Geometry check sheet. Reference: the model listing, model coordinates, mm. Face numbers are marked on the shaded views. A direction names the side the tool comes from. Give positions to 0.01 mm unless a question says otherwise; leave off trailing zeros. Write each loop counter-clockwise with the first axis right and the second up, starting at its lowest first coordinate (ties: lowest second). Pieces come first, ordered by that corner, then holes. Notation, with made-up numbers: (14.5, -34.75) -> (19.5, -34.75) arc R7 cw to (19.5, -22.75) -> close; hole circle Ø3 at (-30.75, 54.5). An arc over 180 degrees is marked (long way). Write item = value, one per line. Start each with the question number.
1. Depth check by flat-ended pin: P1, Ø6.5, axis at x = 325, z = -258.5, coming from the -Y side; P2, Ø11, axis at x = 292.5, z = 7.5, coming from the -Y side; P3, Ø8, axis at x = 92.5, z = 7.5, coming from the +Y side; P4, Ø1, axis at y = 1, z = 300.5, coming from the +X side. Enter the tip coordinate at first touch or a pass-through.
2. Thickness scan on line 1 along X through (y, z) = (1.4, -162.5); line 2 along Z through (x, y) = (-325, 1.55); line 3 along X through (y, z) = (-3.75, 85). Record the ranges inside material, lowest first.
3. Cross-section at B-B, the plane z = -92. Record the cut outline in (x, y).
4. Set-up check for the marked faces 1 and 2: record each of +Z, -Z, +X, -X, +Y, -Y from which the full face is reachable in a straight line by a thin tool's end or side.
5. Cross-section at A-A, the plane y = -6.25. Record the cut outline in (x, z).
6. Cross-section at C-C, the plane x = -145.5. Record the cut outline in (y, z), plus the area to 3 significant figures.
```python
from build123d import *

# Parameters (mm, degrees)
SM_BASE_FLANGE_1_DEPTH = 308.5
SKETCH_6_W             = 10
SKETCH_6_H             = 10
CUT_EXTRUDE_1_DEPTH    = 474.827500257
OTHER_1_DEPTH          = 2
SKETCH_7_R             = 5.5
CUT_EXTRUDE_2_DEPTH    = 10
SKETCH_8_R             = 3.5
CUT_EXTRUDE_3_DEPTH    = 10


# Read off the part's stored shape, not the designer's step: Затупленный угол1
# Sheet-metal steps are written as plain solids
with BuildPart() as part:
    # Sketch 1 → Базовая кромка1 (new, symmetric)
    with BuildSketch(Plane.XY):
        with BuildLine():
            Line((-357.5, -8), (-357.5, -2))
            ThreePointArc((-357.5, -2), (-356.914213562, -0.585786438), (-355.5, 0))
            Line((-355.5, 0), (355.5, 0))
            ThreePointArc((355.5, 0), (356.914213562, -0.585786438), (357.5, -2))
            Line((357.5, -2), (357.5, -8))
            Line((357.5, -8), (359.5, -8))
            Line((359.5, -8), (359.5, -2))
            ThreePointArc((359.5, -2), (358.328427125, 0.828427125), (355.5, 2))
            Line((355.5, 2), (-355.5, 2))
            ThreePointArc((-355.5, 2), (-358.328427125, 0.828427125), (-359.5, -2))
            Line((-359.5, -2), (-359.5, -8))
            Line((-359.5, -8), (-357.5, -8))
        make_face()
    extrude(amount=SM_BASE_FLANGE_1_DEPTH, both=True)

    # Эскиз6 → Вырез-Вытянуть1 (cut, through all)
    with BuildSketch(Plane(origin=(0, 2, 0), x_dir=(1, 0, 0), z_dir=(0, 1, 0))):
        with Locations((-354.5, -303.5)):
            Rectangle(SKETCH_6_W, SKETCH_6_H)
        with Locations((354.5, -303.5)):
            Rectangle(SKETCH_6_W, SKETCH_6_H)
    extrude(amount=-CUT_EXTRUDE_1_DEPTH, mode=Mode.SUBTRACT)

    # Other 1 outline → Other 1 (cut)
    with BuildSketch(Plane(origin=(0, 0, 0), x_dir=(1, 0, 0), z_dir=(0, 1, 0))):
        Polygon((-349.5, -308.5), (-344.5, -308.5), (-349.5, -303.5), align=None)
        Polygon((349.5, -303.5), (344.5, -308.5), (349.5, -308.5), align=None)
    extrude(amount=OTHER_1_DEPTH, mode=Mode.SUBTRACT)

    # Эскиз7 → Вырез-Вытянуть2 (cut)
    with BuildSketch(Plane(origin=(0, 2, 0), x_dir=(1, 0, 0), z_dir=(0, 1, 0))):
        with Locations(Location((325, -293.5, 0), (0, 0, 270))):
            Circle(SKETCH_7_R)
        with Locations(Location((-325, -293.5, 0), (0, 0, 270))):
            Circle(SKETCH_7_R)
        with Locations(Location((-325, 258.5, 0), (0, 0, 270))):
            Circle(SKETCH_7_R)
        with Locations(Location((325, 258.5, 0), (0, 0, 270))):
            Circle(SKETCH_7_R)
    extrude(amount=-CUT_EXTRUDE_2_DEPTH, mode=Mode.SUBTRACT)

    # Эскиз8 → Вырез-Вытянуть3 (cut)
    with BuildSketch(Plane(origin=(0, 2, 0), x_dir=(1, 0, 0), z_dir=(0, 1, 0))):
        with Locations(Location((292.5, 162.5, 0), (0, 0, 270))):
            Circle(SKETCH_8_R)
        with Locations(Location((92.5, 162.5, 0), (0, 0, 270))):
            Circle(SKETCH_8_R)
        with Locations(Location((-107.5, 162.5, 0), (0, 0, 270))):
            Circle(SKETCH_8_R)
        with Locations(Location((-307.5, 162.5, 0), (0, 0, 270))):
            Circle(SKETCH_8_R)
        with Locations(Location((92.5, -7.5, 0), (0, 0, 270))):
            Circle(SKETCH_8_R)
        with Locations(Location((-107.5, -7.5, 0), (0, 0, 270))):
            Circle(SKETCH_8_R)
        with Locations(Location((-307.5, -7.5, 0), (0, 0, 270))):
            Circle(SKETCH_8_R)
        with Locations(Location((92.5, -177.5, 0), (0, 0, 270))):
            Circle(SKETCH_8_R)
        with Locations(Location((-107.5, -177.5, 0), (0, 0, 270))):
            Circle(SKETCH_8_R)
        with Locations(Location((-307.5, -177.5, 0), (0, 0, 270))):
            Circle(SKETCH_8_R)
        with Locations(Location((292.5, -7.5, 0), (0, 0, 270))):
            Circle(SKETCH_8_R)
        with Locations(Location((292.5, -177.5, 0), (0, 0, 270))):
            Circle(SKETCH_8_R)
    extrude(amount=-CUT_EXTRUDE_3_DEPTH, mode=Mode.SUBTRACT)


solid = part.part
```
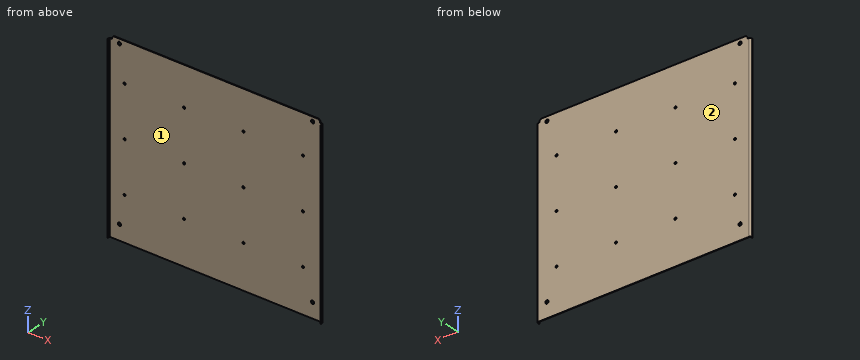
Answers:
q1.P1 = through
q1.P2 = 0
q1.P3 = 2
q1.P4 = 349.5
q2.line_1 = -357.61 to -311, -304 to -111, -104 to 89, 96 to 289, 296 to 357.61
q2.line_2 = -308.5 to -264, -253 to 288, 299 to 308.5
q2.line_3 = -359.5 to -357.5, 357.5 to 359.5
q3.outline = (-359.5, -8) -> (-357.5, -8) -> (-357.5, -2) arc R2 cw to (-355.5, 0) -> (355.5, 0) arc R2 cw to (357.5, -2) -> (357.5, -8) -> (359.5, -8) -> (359.5, -2) arc R4 ccw to (355.5, 2) -> (-355.5, 2) arc R4 ccw to (-359.5, -2) -> close
q4.face_1 = +Z, -Z, -Y
q4.face_2 = +Z, -Z, +X, -X, +Y
q5.outline = (-359.5, -308.5) -> (-357.5, -308.5) -> (-357.5, 298.5) -> (-359.5, 298.5) -> close; (357.5, -308.5) -> (359.5, -308.5) -> (359.5, 298.5) -> (357.5, 298.5) -> close
q6.outline = (0, -308.5) -> (2, -308.5) -> (2, 308.5) -> (0, 308.5) -> close
q6.area = 1,230 mm^2
